Source: CAD feature listing. Evaluate the final solid. Frame: model axes, mm. A direction names the side the tool comes from. Round coordinates to 2 decimals unless told otherwise and drop trailing zeros. Loops run counter-clockwise (first coordinate to the right, second up) from the corner with the lowest first, then second, coordinate; pieces in that order, holes last. Notation, with made-up numbers: (85, 38.5) - (106, 38.5) arc R22 ccw to (106, 70.5) - close; hole circle Ø4 at (22, -24.75). An arc over 180 degrees is marked (long way). One line per question, with ' | ' between items.
from build123d import *

# Parameters (mm, degrees)
F1_DEPTH = 247.65
F2_R     = 63.5
F3_DEPTH = 48.261
F2_W     = 254
F2_H     = 127
F4_DEPTH = 48.261
F5_R     = 38.1
F6_DEPTH = 218.44
F7_DEPTH = 218.44
F8_R     = 127


with BuildPart() as f1:
    # F0 (on Front) → F1 (new body, symmetric)
    with BuildSketch(Plane.XZ):
        with BuildLine():
            ThreePointArc((-712.5918887531, 174.2182937558), (-718.5813490984, 59.272102872), (-619.9136327213, 0))
            Line((-619.9136327213, 0), (650.0863672787, 0))
            Line((650.0863672787, 0), (650.0863672787, 48.26))
            Line((650.0863672787, 48.26), (-619.9136327213, 48.26))
            ThreePointArc((-619.9136327213, 48.26), (-675.0054873243, 80.18251504), (-674.7061432771, 143.8540927118))
            Line((-674.7061432771, 143.8540927118), (-229.4541094396, 589.1061265492))
            Line((-229.4541094396, 589.1061265492), (-263.5790826997, 623.2310998093))
            Line((-263.5790826997, 623.2310998093), (-712.5918887531, 174.2182937558))
        make_face()
    extrude(amount=F1_DEPTH, both=True)

    # F2 (on face) → F3 (cut, through all)
    with BuildSketch(Plane.XY.offset(48.26)):
        with Locations((-162.7136327213, 0)):
            Circle(F2_R)
    extrude(amount=-F3_DEPTH, mode=Mode.SUBTRACT)

    # F2 (on face) → F4 (cut, through all)
    with BuildSketch(Plane.XY.offset(48.26)):
        with Locations((354.1763672787, 0)):
            Rectangle(F2_W, F2_H)
        with BuildLine():
            ThreePointArc((227.1763672787, 63.5), (163.6763672787, 0), (227.1763672787, -63.5))
            Line((227.1763672787, -63.5), (227.1763672787, 63.5))
        make_face()
        with BuildLine():
            Line((481.1763672787, 63.5), (481.1763672787, -63.5))
            ThreePointArc((481.1763672787, -63.5), (544.6763672787, 0), (481.1763672787, 63.5))
        make_face()
    extrude(amount=-F4_DEPTH, mode=Mode.SUBTRACT)

    # F5 (on face) → F6 (cut)
    with BuildSketch(Plane(origin=(-443.4050912545, 0, 443.4050912545), x_dir=(0, -1, 0), z_dir=(-0.7071067812, 0, 0.7071067812))):
        with Locations((133.35, 25.7123801656)):
            Circle(F5_R)
    extrude(amount=-F6_DEPTH, mode=Mode.SUBTRACT)

    # F5 (on face) → F7 (cut)
    with BuildSketch(Plane(origin=(-443.4050912545, 0, 443.4050912545), x_dir=(0, -1, 0), z_dir=(-0.7071067812, 0, 0.7071067812))):
        with Locations((-133.35, 25.7123801656)):
            Circle(F5_R)
    extrude(amount=-F7_DEPTH, mode=Mode.SUBTRACT)

    # F8
    f8_edges = [f1.edges().sort_by_distance(p)[0] for p in [
        (650.086367, -247.65, 24.13),
        (650.086367, 247.65, 24.13),
        (-246.516596, -247.65, 606.168613),
        (-246.516596, 247.65, 606.168613),
    ]]
    fillet(f8_edges, radius=F8_R)


solid = f1.part
1. Material intervals for probe 1 along Y at (x, z) = (471, 40); probe 2 along Z at (x, y) = (197.5, -116.5); probe 3 along Z at (x, y) = (-237.5, 127), sorted ascending.
Worked out:
probe 1: y = -247.65 to -63.5, 63.5 to 247.65 | probe 2: z = 0 to 48.26 | probe 3: z = 0 to 48.26, 581.06 to 596.93
2. Section query A-A, the plane x = 416.5. Return loops of the section in (y, z).
Worked out:
outline: (-247.65, 0) - (-63.5, 0) - (-63.5, 48.26) - (-247.65, 48.26) - close; (63.5, 0) - (247.65, 0) - (247.65, 48.26) - (63.5, 48.26) - close
3. Section query B-B, the plane y = 0. Return loops of the section in (x, z).
Worked out:
outline: (-712.59, 174.22) arc R111.76 ccw to (-619.91, 0) - (-226.21, 0) - (-226.21, 48.26) - (-619.91, 48.26) arc R63.5 cw to (-674.71, 143.85) - (-229.45, 589.11) - (-263.58, 623.23) - close; (-99.21, 0) - (163.68, 0) - (163.68, 48.26) - (-99.21, 48.26) - close; (544.68, 0) - (650.09, 0) - (650.09, 48.26) - (544.68, 48.26) - close
4. Access query for faces 4 (the flat face through (352, -63.5, 24)), 5 (the flat face through (-455.2, -3.47, 363.36)), 6 (the cylindrical face through (611.9, -211.43, 24.47)). Directions: +Z, -Z, +X, -X, +Y, -Y. A direction counts if a zero-diameter tool reaches every point of the face in a straight line with its end or side. Return the directions, or none.
Worked out:
face 4: +Z, -Z | face 5: +X, +Y, -Y | face 6: +Z, -Z, +X, -Y
5. Section query D-D, the plane x = 129. Return loops of the section in (y, z).
Worked out:
outline: (-247.65, 0) - (247.65, 0) - (247.65, 48.26) - (-247.65, 48.26) - close
6. Contact query for flat-ended pins moving along their axis: P1, Ø8, axis at x = -60.5, y = 84.5, coming from the -Z side; P2, Ø1.5, axis at x = -73, y = 110, coming from the +Z side; P3, Ø12, axis at x = -508, y = 48, coming from the +Z side. Output: stop coordinate, or through.
Worked out:
P1: stops at z = 0 | P2: stops at z = 48.26 | P3: stops at z = 384.81
7. Mould query, pull axis X, two halves, no side actions, for faces 1 (the cylindrical face through (-424.793, 163.585, 428.37)), 2 (the flat face through (-293, -247.65, 31)), 3 (the flat face through (-246.28, -1.69, 605.93)). Classes: released by +X, released by -X, zero draft, split by the parting line, or undercut.
Worked out:
face 1: undercut | face 2: zero draft | face 3: released by +X
8. Section query C-C, the plane y = -140. Return loops of the section in (x, z), plus the area to 3 significant figures.
Worked out:
outline: (-712.59, 174.22) arc R111.76 ccw to (-619.91, 0) - (648.6, 0) - (648.6, 48.26) - (-619.91, 48.26) arc R63.5 cw to (-674.71, 143.85) - (-417.63, 400.93) - (-451.75, 435.06) - close; (-398.7, 488.11) - (-364.57, 453.99) - (-230.5, 588.06) - (-264.63, 622.18) - close | area: 97,100 mm2
